Read the model definition and answer for the solid it produces. Units are mm, in the model's axes. Coordinates: 2 decimals unless noted, no trailing zeros. Write each loop counter-clockwise with the first axis right and the second up, starting at its lowest first coordinate (ties: lowest second). Pieces come first, ordered by that corner, then holes. Notation, with made-up numbers: (-10.5, -29) - (25.5, -29) arc R28 ccw to (25.5, 8) - close; hole circle Ø10 at (40.25, -37.5). An arc over 180 degrees is marked (long way). Use a Markdown table: item, result.
from build123d import *

# Parameters (mm, degrees)
F2_DEPTH = 6.35
F1_R     = 3.175
F3_DEPTH = 6.351


with BuildPart() as f2:
    # F0 (on Top) → F2 (new body)
    with BuildSketch(Plane.XY):
        with BuildLine():
            Line((9.545455, 0), (62.045455, 0))
            ThreePointArc((62.045455, 0), (72.045455, 10), (62.045455, 20))
            Line((62.045455, 20), (9.545455, 20))
            ThreePointArc((9.545455, 20), (-0.454545, 10), (9.545455, 0))
        make_face()
    extrude(amount=F2_DEPTH)

    # F1 (on face) → F3 (cut, through all)
    with BuildSketch(Plane.XY):
        with Locations((62.045455, 10)):
            Circle(F1_R)
        with Locations((9.545455, 10)):
            Circle(F1_R)
    extrude(amount=F3_DEPTH, mode=Mode.SUBTRACT)


solid = f2.part
(1) Each of these flat-tipped pins is pushed along its axis until it touches: P1, Ø4, axis at x = 13.5, y = 14.5, coming from the -Z side; P2, Ø1.5, axis at y = 13, z = 2, coming from the +X side. Where does it stop, or does it pass through?
Report:
| item | result |
|---|---|
| P1 | stops at z = 0 |
| P2 | stops at x = 71.79 |
(2) The mould has two halves that part along X. Classify faces 1 (the cylindrical face through (72.043, 9.78, 3.131)), 2 (the cylindrical face through (64.978, 8.784, 3.131)), 3 (the flat face through (35, 10, 0)): pulls with the +X half, pulls with the -X half, needs draft (parallel to the pull), parting line crosses it, or undercut.
Report:
| item | result |
|---|---|
| face 1 | pulls with the +X half |
| face 2 | undercut |
| face 3 | needs draft |
(3) A cutting plane is placed at B-B, the plane z = 4.75. Write down the section's boundary in (x, y) (3 decimals), and give its area (3 significant figures).
Report:
| item | result |
|---|---|
| outline | (9.545, 0) - (62.045, 0) arc R10 ccw to (62.045, 20) - (9.545, 20) arc R10 ccw to start; hole circle Ø6.35 at (9.545, 10); hole circle Ø6.35 at (62.045, 10) |
| area | 1,300 mm² |
(4) A cutting plane is placed at D-D, the plane x = 67. Write down the section's boundary in (y, z).
Report:
| item | result |
|---|---|
| outline | (1.31, 0) - (18.69, 0) - (18.69, 6.35) - (1.31, 6.35) - close |
(5) Straight lines are drawn through the part: L1, parallel to X at y = 10, z = 3.25; L2, parallel to X at y = 8.25, z = 6; L3, parallel to Y at x = 63.5, z = 1. For each, find the intervals that lie inside material, in ascending order.
Report:
| item | result |
|---|---|
| L1 | x = -0.45 to 6.37, 12.72 to 58.87, 65.22 to 72.05 |
| L2 | x = -0.3 to 6.9, 12.19 to 59.4, 64.69 to 71.89 |
| L3 | y = 0.11 to 7.18, 12.82 to 19.89 |
(6) A cutting plane is placed at A-A, the plane y = 10. Write down the section's boundary in (x, z), and give its area (3 significant figures).
Report:
| item | result |
|---|---|
| outline | (-0.45, 0) - (6.37, 0) - (6.37, 6.35) - (-0.45, 6.35) - close; (12.72, 0) - (58.87, 0) - (58.87, 6.35) - (12.72, 6.35) - close; (65.22, 0) - (72.05, 0) - (72.05, 6.35) - (65.22, 6.35) - close |
| area | 380 mm² |
(7) A cutting plane is placed at C-C, the plane y = 16.5. Write down the section's boundary in (x, z).
Report:
| item | result |
|---|---|
| outline | (1.95, 0) - (69.64, 0) - (69.64, 6.35) - (1.95, 6.35) - close |
